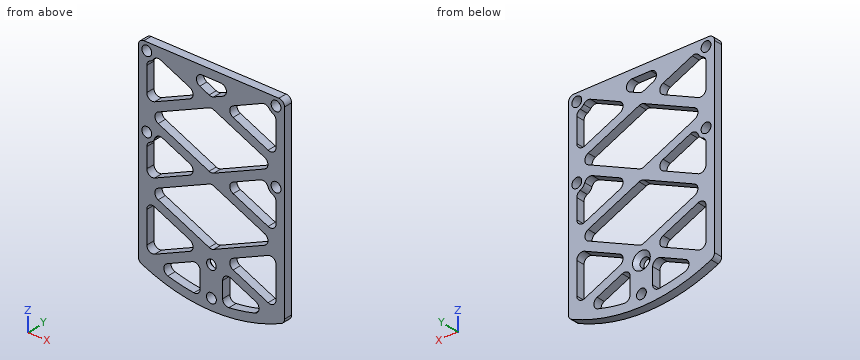
```python
from build123d import *

# Parameters (mm, degrees)
BOSS_EXTRUDE1_DEPTH = 3
SKETCH2_R           = 1.75
CUT_EXTRUDE1_DEPTH  = 66.459911396
SKETCH3_R           = 1.75
CUT_EXTRUDE2_DEPTH  = 66.459911396
CUT_EXTRUDE3_DEPTH  = 66.459911396
FILLET1_R           = 2


with BuildPart() as part:
    # Sketch1 → Boss-Extrude1 (new body)
    with BuildSketch(Plane(origin=(0, 0, 0), x_dir=(1, 0, 0), z_dir=(0, 1, 0))):
        with BuildLine():
            Line((-26, -15.8), (26, -15.8))
            Line((26, -15.8), (26, 54.074023338))
            ThreePointArc((26, 54.074023338), (0, 60), (-26, 54.074023338))
            Line((-26, 54.074023338), (-26, -15.8))
        make_face()
    extrude(amount=BOSS_EXTRUDE1_DEPTH)

    # Sketch2 → Cut-Extrude1 (cut, through all)
    with BuildSketch(Plane(origin=(0, 3, 0), x_dir=(1, 0, 0), z_dir=(0, 1, 0))):
        with Locations(Location((-23, -13, 0), (0, 0, 270))):
            Circle(SKETCH2_R)
        with Locations(Location((-23, 12.5, 0), (0, 0, 270))):
            Circle(SKETCH2_R)
        with Locations(Location((23, -13, 0), (0, 0, 270))):
            Circle(SKETCH2_R)
        with Locations(Location((23, 12.5, 0), (0, 0, 270))):
            Circle(SKETCH2_R)
    extrude(amount=-CUT_EXTRUDE1_DEPTH, mode=Mode.SUBTRACT)

    # Sketch3 → Cut-Extrude2 (cut, through all)
    with BuildSketch(Plane(origin=(0, 3, 0), x_dir=(1, 0, 0), z_dir=(0, 1, 0))):
        with Locations(Location((0, 56, 0), (0, 0, 270))):
            Circle(SKETCH3_R)
    extrude(amount=-CUT_EXTRUDE2_DEPTH, mode=Mode.SUBTRACT)

    # Sketch4 → Cut-Extrude3 (cut, through all)
    with BuildSketch(Plane(origin=(0, 3, 0), x_dir=(1, 0, 0), z_dir=(0, 1, 0))):
        with BuildLine():
            Line((-4, 56.859475903), (-4, 45.835789761))
            Line((-4, 45.835789761), (-20.43478188, 53.211086152))
            ThreePointArc((-20.43478188, 53.211086152), (-12.352826734, 55.645374216), (-4, 56.859475903))
        make_face()
        with BuildLine():
            Line((4, 56.859475903), (4, 45.835789761))
            Line((4, 45.835789761), (20.43478188, 53.211086152))
            ThreePointArc((20.43478188, 53.211086152), (12.352826734, 55.645374216), (4, 56.859475903))
        make_face()
        Polygon((-23, 51.074023338), (-3.66367684, 42.396627103), (-23, 33.719230867), align=None)
        Polygon((3.66367684, 42.396627103), (23, 51.074023338), (23, 33.719230867), align=None)
        Polygon((0, 40.752510206), (-23, 30.430997074), (0, 20.109483942), (23, 30.430997074), align=None)
        with BuildLine():
            Line((-23, 27.142763282), (-3.66367684, 18.465367046))
            Line((-3.66367684, 18.465367046), (-20.439245255, 10.937138798))
            ThreePointArc((-20.439245255, 10.937138798), (-20.383840257, 13.968233019), (-23, 15.5))
            Line((-23, 15.5), (-23, 27.142763282))
        make_face()
        with BuildLine():
            Line((3.66367684, 18.465367046), (23, 27.142763282))
            Line((23, 27.142763282), (23, 15.5))
            ThreePointArc((23, 15.5), (20.383840257, 13.968233019), (20.439245255, 10.937138798))
            Line((20.439245255, 10.937138798), (3.66367684, 18.465367046))
        make_face()
        Polygon((0, 16.821250149), (-23, 6.499737017), (0, -3.821776115), (23, 6.499737017), align=None)
        with BuildLine():
            Line((23, 3.211503225), (3.66367684, -5.465893011))
            Line((3.66367684, -5.465893011), (20.006674091, -12.8))
            ThreePointArc((20.006674091, -12.8), (20.950609847, -10.80910977), (23, -10))
            Line((23, -10), (23, 3.211503225))
        make_face()
        with BuildLine():
            Line((-23, -10), (-23, 3.211503225))
            Line((-23, 3.211503225), (-3.66367684, -5.465893011))
            Line((-3.66367684, -5.465893011), (-20.006674091, -12.8))
            ThreePointArc((-20.006674091, -12.8), (-20.950609847, -10.80910977), (-23, -10))
        make_face()
        Polygon((-12.679320411, -12.8), (0, -7.110009907), (12.679320411, -12.8), align=None)
    extrude(amount=-CUT_EXTRUDE3_DEPTH, mode=Mode.SUBTRACT)

    # Fillet1
    fillet1_edges = [part.edges().sort_by_distance(p)[0] for p in [
        (20.439245255, 1.5, -10.937138798),
        (3.66367684, 1.5, -18.465367046),
        (23, 1.5, -27.142763282),
        (23, 1.5, -15.5),
        (0, 1.5, -16.821250149),
        (23, 1.5, -6.499737017),
        (0, 1.5, 3.821776115),
        (-23, 1.5, -6.499737017),
        (23, 1.5, -3.211503225),
        (23, 1.5, 10),
        (20.006674091, 1.5, 12.8),
        (3.66367684, 1.5, 5.465893011),
        (-20.006674091, 1.5, 12.8),
        (-23, 1.5, 10),
        (-23, 1.5, -3.211503225),
        (-3.66367684, 1.5, 5.465893011),
        (12.679320411, 1.5, 12.8),
        (-12.679320411, 1.5, 12.8),
        (0, 1.5, 7.110009907),
        (4, 1.5, -56.859475903),
        (20.43478188, 1.5, -53.211086152),
        (4, 1.5, -45.835789761),
        (-20.43478188, 1.5, -53.211086152),
        (-4, 1.5, -56.859475903),
        (-4, 1.5, -45.835789761),
        (-23, 1.5, -33.719230867),
        (-23, 1.5, -51.074023338),
        (-3.66367684, 1.5, -42.396627103),
        (23, 1.5, -33.719230867),
        (3.66367684, 1.5, -42.396627103),
        (23, 1.5, -51.074023338),
        (-26, 1.5, -54.074023338),
        (26, 1.5, -54.074023338),
        (26, 1.5, 15.8),
        (-26, 1.5, 15.8),
        (0, 1.5, -40.752510206),
        (23, 1.5, -30.430997074),
        (0, 1.5, -20.109483942),
        (-23, 1.5, -30.430997074),
        (-23, 1.5, -15.5),
        (-23, 1.5, -27.142763282),
        (-3.66367684, 1.5, -18.465367046),
        (-20.439245255, 1.5, -10.937138798),
    ]]
    fillet(fillet1_edges, radius=FILLET1_R)

    # Sketch5 → CSK for M3 Countersunk Flat Head Screw1 (revolve, cut)
    with BuildSketch(Plane(origin=(0, 3, -45.5), x_dir=(0, 0, 1), z_dir=(1, 0, 0))):
        Polygon((0, 0), (0, 3), (1.7, 3), (1.7, 1.45), (3.15, 0), align=None)
    revolve(axis=Axis((0, 9.35, -45.5), (0, -1, 0)), mode=Mode.SUBTRACT)


solid = part.part
```
Read the model definition and answer for the solid it produces. Units are mm, in the model's axes. Round coordinates to 2 decimals unless told otherwise and drop trailing zeros. Write each loop counter-clockwise with the first axis right and the second up, starting at its lowest first coordinate (ties: lowest second). Pieces come first, ordered by that corner, then holes. Notation, with made-up numbers: (-4.5, 75) -> (15.5, 75) arc R17 ccw to (15.5, 82) -> close; hole circle Ø10 at (7.25, 68). An arc over 180 degrees is marked (long way). Answer in a Markdown table with one row per item. Add a question column.
1) Consider line 1 (X direction, y = 1.2, z = 13); line 2 (X direction, y = 1.8, z = -0.5); line 3 (X direction, y = 2.3, z = -25). Determine where each line is inside the solid, lowest interval first.
2) Find section A-A, the plane x = 0. Determine the outline of the cut face in (y, z), and give its area (3 significant figures).
3) Find section B-B, the plane z = -45.5. Determine the outline of the cut face in (x, y).
4) Given P1, Ø3, axis at x = 0, z = -45.5, coming from the -Y side; P2, Ø1.5, axis at x = 0, y = 2, coming from the -Z side, each flat-ended and moving along its own axis, determine where each tip first touches the part or whether it passes through.
5) Find section C-C, the plane y = 2.25. State how many separate pieces and enclosed holes the cut face has, and give its area (3 significant figures).
6) Find section D-D, the plane z = -21.5. Determine the outline of the cut face in (x, y).
Findings below:
| question | item | result |
|---|---|---|
| 1 | line 1 | -26 to -24.75, -21.25 to 21.25, 24.75 to 26 |
| 1 | line 2 | -26 to -22.96, -16.96 to -9.63, 9.63 to 16.96, 22.96 to 26 |
| 1 | line 3 | -26 to -22.76, -18.23 to -10.9, 10.9 to 18.23, 22.76 to 26 |
| 2 | outline | (0, -60) -> (3, -60) -> (3, -57.75) -> (0, -57.75) -> close; (0, -54.25) -> (3, -54.25) -> (3, -48.65) -> (1.55, -47.2) -> (0, -47.2) -> close; (0, -43.8) -> (1.55, -43.8) -> (3, -42.35) -> (3, -40.56) -> (0, -40.56) -> close; (0, -20.3) -> (3, -20.3) -> (3, -16.63) -> (0, -16.63) -> close; (0, 3.63) -> (3, 3.63) -> (3, 7.3) -> (0, 7.3) -> close; (0, 12.8) -> (3, 12.8) -> (3, 15.8) -> (0, 15.8) -> close |
| 2 | area | 66.6 mm² |
| 3 | outline | (-26, 0) -> (-23, 0) -> (-23, 3) -> (-26, 3) -> close; (-10.58, 0) -> (-1.7, 0) -> (-1.7, 1.55) -> (-3.15, 3) -> (-10.58, 3) -> close; (1.7, 0) -> (10.58, 0) -> (10.58, 3) -> (3.15, 3) -> (1.7, 1.55) -> close; (23, 0) -> (26, 0) -> (26, 3) -> (23, 3) -> close |
| 4 | P1 | through |
| 4 | P2 | z = -60 |
| 5 | separate pieces | 1 |
| 5 | enclosed holes | 17 |
| 5 | area | 1,700 mm² |
| 6 | outline | (-26, 0) -> (-23, 0) -> (-23, 3) -> (-26, 3) -> close; (-10.43, 0) -> (-3.1, 0) -> (-3.1, 3) -> (-10.43, 3) -> close; (3.1, 0) -> (10.43, 0) -> (10.43, 3) -> (3.1, 3) -> close; (23, 0) -> (26, 0) -> (26, 3) -> (23, 3) -> close |
